```python
from build123d import *

# Parameters (mm, degrees)
F0_W      = 53
F0_H      = 53
F1_DEPTH  = 60
F3_DEPTH  = 4
F4_DEPTH  = 53
F6_DEPTH  = 6
F8_DEPTH  = 60
F10_DEPTH = 4
F9_W      = 60
F9_H      = 10
F11_DEPTH = 10
F12_DEPTH = 25


with BuildPart() as f1:
    # F0 (on Right) → F1 (new body)
    with BuildSketch(Plane.YZ):
        with Locations((26.5, 26.5)):
            Rectangle(F0_W, F0_H)
    extrude(amount=F1_DEPTH)

    # F2 (on face) → F3 (cut)
    with BuildSketch(Plane.XY.offset(53)):
        with BuildLine():
            ThreePointArc((9.5867410065, 49.0510278539), (3.9489721461, 48.5867410065), (4.4132589935, 42.9489721461))
            Line((4.4132589935, 42.9489721461), (27.4132590282, 23.4489721167))
            ThreePointArc((27.4132590282, 23.4489721167), (26, 26.4999999772), (27.4132589935, 29.5510278539))
            Line((27.4132589935, 29.5510278539), (30, 31.7441343594))
            Line((30, 31.7441343594), (9.5867410065, 49.0510278539))
        make_face()
        with BuildLine():
            ThreePointArc((32.5867410065, 23.4489721461), (30.0000000228, 22.5), (27.4132590282, 23.4489721167))
            Line((27.4132590282, 23.4489721167), (50.4132589935, 3.9489721461))
            ThreePointArc((50.4132589935, 3.9489721461), (56.0510278539, 4.4132589935), (55.5867410065, 10.0510278539))
            Line((55.5867410065, 10.0510278539), (36.1853892444, 26.5))
            Line((36.1853892444, 26.5), (32.5867410065, 23.4489721461))
        make_face()
        with BuildLine():
            ThreePointArc((27.4132589935, 29.5510278539), (26, 26.4999999772), (27.4132590282, 23.4489721167))
            ThreePointArc((27.4132590282, 23.4489721167), (30.0000000228, 22.5), (32.5867410065, 23.4489721461))
            Line((32.5867410065, 23.4489721461), (36.1853892444, 26.5))
            Line((36.1853892444, 26.5), (55.5867410065, 42.9489721461))
            ThreePointArc((55.5867410065, 42.9489721461), (56.0510278539, 48.5867410065), (50.4132589935, 49.0510278539))
            Line((50.4132589935, 49.0510278539), (30, 31.7441343594))
            Line((30, 31.7441343594), (27.4132589935, 29.5510278539))
        make_face()
        with BuildLine():
            ThreePointArc((16, 29), (12, 33), (8, 29))
            Line((8, 29), (8, 12))
            ThreePointArc((8, 12), (9.1715728753, 9.1715728753), (12, 8))
            Line((12, 8), (29, 8))
            ThreePointArc((29, 8), (33, 12), (29, 16))
            Line((29, 16), (16, 16))
            Line((16, 16), (16, 29))
        make_face()
    extrude(amount=-F3_DEPTH, mode=Mode.SUBTRACT)

    # F2 (on face) → F4 (cut, through all)
    with BuildSketch(Plane.XY.offset(53)):
        Polygon((38.48, 53), (21.52, 53), (30, 44.52), align=None)
    extrude(amount=-F4_DEPTH, mode=Mode.SUBTRACT)

    # F5 (on face) → F6 (cut)
    with BuildSketch(Plane.XZ):
        Polygon((27.1889083829, 53), (12.0839592813, 53), (60, 10.6741640318), (60, 24.0168690716), align=None)
        Polygon((47.9160407187, 0), (0, 42.3258359682), (0, 28.9831309284), (32.8110916171, 0), align=None)
    extrude(amount=-F6_DEPTH, mode=Mode.SUBTRACT)

    # F7 (on face) → F8 (cut, through all)
    with BuildSketch(Plane(origin=(0, 0, 0), x_dir=(0, -1, 0), z_dir=(-1, 0, 0))):
        Polygon((-44.52, 26.5), (-53, 34.98), (-53, 18.02), align=None)
    extrude(amount=-F8_DEPTH, mode=Mode.SUBTRACT)

    # F9 (on face) → F10 (cut)
    with BuildSketch(Plane(origin=(0, 0, 0), x_dir=(1, 0, 0), z_dir=(0, 0, -1))):
        Polygon((0, -16), (60, -16), (60, -4), (47.9160407187, -4), (47.9160407187, -6), (32.8110916171, -6), (32.8110916171, -4), (0, -4), align=None)
        Polygon((38.48, -53), (60, -53), (60, -45), (30.48, -45), align=None)
    extrude(amount=-F10_DEPTH, mode=Mode.SUBTRACT)

    # F9 (on face) → F11 (cut)
    with BuildSketch(Plane(origin=(0, 0, 0), x_dir=(1, 0, 0), z_dir=(0, 0, -1))):
        with Locations((30, -30)):
            Rectangle(F9_W, F9_H)
    extrude(amount=-F11_DEPTH, mode=Mode.SUBTRACT)

    # F12 (cut): a face of the model
    f12_faces = [f1.faces().sort_by_distance(p)[0] for p in [
        (47.9160407187, 5, 2),
    ]]
    extrude(f12_faces, amount=-F12_DEPTH, mode=Mode.SUBTRACT)


solid = f1.part
```
CAD build for the part. Positions are in the model's coordinates, mm. A direction names the side the tool comes from. Round coordinates to 2 decimals unless told otherwise and drop trailing zeros. Write each loop counter-clockwise with the first axis right and the second up, starting at its lowest first coordinate (ties: lowest second). Pieces come first, ordered by that corner, then holes. Notation, with made-up numbers: (-0.5, -27) - (26.5, -27) arc R22 cw to (26.5, -7) - close; hole circle Ø11 at (85, 25.25). An arc over 180 degrees is marked (long way). Write item = value, one per line. Start each with the question number.
Q1. Band-saw the part on B-B (z = 39). Give the cut face in (x, y), then the cut area to 3 significant figures.
Q2. Band-saw the part on A-A (y = 47). Give the cut face in (x, z), then the cut area to 3 significant figures.
Q3. Which spindle directions (+Z, -Z, +X, -X, +Y, -Y) get a long thin tool onto all of the face, cutting with end or side? Do faces 3 (the flat face through (11.46, 48.7, 30.68)), 4 (the flat face through (45, 45, 2)), 5 (the flat face through (8, 21, 51)), 6 (the flat face through (24.29, 2.96, 20.87)), 7 (the flat face through (34.18, 48.7, 13.44)). Say none if no direction does.
Q4. Probe L1, parallel to Y at x = 55.5, z = 6; L2, parallel to Y at x = 41.5, z = 51.5; L3, parallel to Z at x = 31, y = 14. List the from-to ranges inside material, lowest first. Write a range as from..to.
Q5. Band-saw the part on D-D (y = 7). Give the cut face in (x, z).
Q6. Band-saw the part on C-C (x = 7). Give the cut face in (y, z), then the cut area to 3 significant figures.
Q7. Drop flat-ended pins along their axis: pin 1 (21 mm diameter, centred on x = 25.5, z = 28, fed in from -Y); pin 2 (1 mm diameter, centred on x = 43.5, z = 28, fed in from +Y); pin 3 (4.5 mm diameter, centred on x = 22, z = 51, fed in from -Y); pin 4 (3 mm diameter, centred on x = 38, z = 2, fed in from +Y). Give the stop position or say it passes through.
Q8. Mould opens along X. For faces 1 (the flat face through (11, 53, 44)), 2 (the cylindrical face through (9.141, 9.203, 51.028)) say: pulls with the +X half, pulls with the -X half, needs draft (parallel to the pull), parting line crosses it, or undercut.
Answers below:
q1.outline = (0, 6) - (3.77, 6) - (3.77, 0) - (27.93, 0) - (27.93, 6) - (43.04, 6) - (43.04, 0) - (60, 0) - (60, 53) - (38.48, 53) - (30, 44.52) - (21.52, 53) - (0, 53) - close
q1.area = 2,990 mm2
q2.outline = (0, 0) - (27.52, 0) - (27.52, 24.02) - (0, 24.02) - close; (0, 28.98) - (27.52, 28.98) - (27.52, 53) - (12.01, 53) - (12.01, 49) - (3.13, 49) - (3.13, 53) - (0, 53) - close; (32.48, 4) - (60, 4) - (60, 24.02) - (32.48, 24.02) - close; (32.48, 28.98) - (60, 28.98) - (60, 53) - (56.87, 53) - (56.87, 49) - (47.99, 49) - (47.99, 53) - (32.48, 53) - close
q2.area = 2,460 mm2
q3.face_3 = +X, -X, +Y
q3.face_4 = -Z, +X, +Y
q3.face_5 = +Z
q3.face_6 = -Y
q3.face_7 = +Z, -Z, +Y
q4.L1 = 0..25, 35..53
q4.L2 = 0..11.51, 21.99..31.01, 41.49..53
q4.L3 = 4..49
q5.outline = (0, 4) - (60, 4) - (60, 53) - (57, 53) - (57, 49) - (46.81, 49) - (46.81, 53) - (0, 53) - close
q6.outline = (0, 0) - (4, 0) - (4, 4) - (16, 4) - (16, 0) - (25, 0) - (25, 10) - (35, 10) - (35, 0) - (53, 0) - (53, 18.02) - (44.52, 26.5) - (53, 34.98) - (53, 53) - (50, 53) - (50, 49) - (40.76, 49) - (40.76, 53) - (0, 53) - (0, 36.14) - (6, 36.14) - (6, 22.8) - (0, 22.8) - close
q6.area = 2,470 mm2
q7.pin_1 = 0
q7.pin_2 = 46.52
q7.pin_3 = 6
q7.pin_4 = 45
q8.face_1 = needs draft
q8.face_2 = undercut
